from build123d import *

# Parameters (mm, degrees)
SKETCH1_W           = 30
SKETCH1_H           = 5
BOSS_EXTRUDE1_DEPTH = 15
SKETCH3_R           = 1
CUT_EXTRUDE2_DEPTH  = 5
SKETCH4_R           = 2
CUT_EXTRUDE3_DEPTH  = 1.5
SKETCH5_W           = 5
SKETCH5_H           = 10
BOSS_EXTRUDE2_DEPTH = 3


with BuildPart() as part:
    # Sketch1 → Boss-Extrude1 (new body)
    with BuildSketch(Plane(origin=(0, 0, 0), x_dir=(1, 0, 0), z_dir=(0, 1, 0))):
        with Locations((-41.880536913, 26.290268456)):
            Rectangle(SKETCH1_W, SKETCH1_H)
    extrude(amount=BOSS_EXTRUDE1_DEPTH)

    # Sketch3 → Cut-Extrude2 (cut)
    with BuildSketch(Plane(origin=(0, 0, -28.790268456), x_dir=(-1, 0, 0), z_dir=(0, 0, -1))):
        with Locations((35.880536913, 7.5)):
            Circle(SKETCH3_R)
        with Locations((32.880536913, 7.5)):
            Circle(SKETCH3_R)
        with Locations((29.880536913, 7.5)):
            Circle(SKETCH3_R)
        with Locations((53.880536913, 7.5)):
            Circle(SKETCH3_R)
        with Locations((50.880536913, 7.5)):
            Circle(SKETCH3_R)
        with Locations((47.880536913, 7.5)):
            Circle(SKETCH3_R)
    extrude(amount=-CUT_EXTRUDE2_DEPTH, mode=Mode.SUBTRACT)

    # Sketch4 → Cut-Extrude3 (cut)
    with BuildSketch(Plane(origin=(0, 0, -28.790268456), x_dir=(-1, 0, 0), z_dir=(0, 0, -1))):
        with Locations((41.880536913, 7.5)):
            Circle(SKETCH4_R)
    extrude(amount=-CUT_EXTRUDE3_DEPTH, mode=Mode.SUBTRACT)

    # Sketch5 → Boss-Extrude2 (add)
    with BuildSketch(Plane.XY.offset(-23.790268456)):
        with Locations((-59.380536913, 7.5)):
            Rectangle(SKETCH5_W, SKETCH5_H)
        with Locations((-24.380536913, 7.5)):
            Rectangle(SKETCH5_W, SKETCH5_H)
    extrude(amount=-BOSS_EXTRUDE2_DEPTH)


solid = part.part
Model file for the job. Use its own axes, mm. A direction names the side the tool comes from. Give positions to 0.01 mm unless a question says otherwise; leave off trailing zeros. Loops run counter-clockwise (first coordinate to the right, second up) from the corner with the lowest first, then second, coordinate; pieces in that order, holes last. Notation, with made-up numbers: (23.25, -26) - (28.25, -26) arc R20 ccw to (28.25, -2) - close; hole circle Ø11 at (-19, 58). An arc over 180 degrees is marked (long way). Use one line per item in the form item = value.
(1) Cut at C-C (y = 3.75). Give the cut face in (x, z), then the cut area to 3 significant figures.
Determined:
outline = (-61.88, -26.79) - (-56.88, -26.79) - (-56.88, -28.79) - (-26.88, -28.79) - (-26.88, -26.79) - (-21.88, -26.79) - (-21.88, -23.79) - (-61.88, -23.79) - close
area = 180 mm^2
(2) Drill centre lines: L1, parallel to X at y = 11.5, z = -27.2; L2, parallel to Y at x = -26, z = -25.1; L3, parallel to Z at x = -57.5, y = 6.5. Where is each one in solid material? Low to high.
Determined:
L1 = -56.88 to -26.88
L2 = 2.5 to 12.5
L3 = -26.79 to -23.79
(3) Pull direction Y, two halves, no side cores. Call faces 1 (the face through (-24, 2.5, -25)), 2 (the face through (-43.79, 8.1, -28.05)), 3 (the face through (-45, 7, -28.79)), 4 (the face through (-49.88, 7.54, -26.33)): pulls with the +Y half, pulls with the -Y half, needs draft (parallel to the pull), parting line crosses it, or undercut.
Determined:
face_1 = pulls with the -Y half
face_2 = undercut
face_3 = needs draft
face_4 = undercut
(4) Cut at D-D (y = 7.5). Count the separate pieces of the cut face and the enclosed holes in it, then the cut area to 3 significant figures.
Determined:
separate_pieces = 7
enclosed_holes = 0
area = 114 mm^2
(5) Cut at B-B (x = -53.5). Give the cut face in (y, z), then the cut area to 3 significant figures.
Determined:
outline = (0, -28.79) - (6.58, -28.79) - (6.58, -23.79) - (0, -23.79) - close; (8.42, -28.79) - (15, -28.79) - (15, -23.79) - (8.42, -23.79) - close
area = 65.8 mm^2
(6) Drop flat-ended pins along their axis: P1, Ø1.5, axis at x = -24.5, z = -25.5, coming from the -Y side; P2, Ø2.5, axis at x = -60, z = -25, coming from the +Y side; P3, Ø1.2, axis at x = -32.88, y = 7.5, coming from the -Z side; P4, Ø1.5, axis at x = -24.5, y = 9.5, coming from the -Z side. Give the stop position or say it passes through.
Determined:
P1 = 2.5
P2 = 12.5
P3 = through
P4 = -26.79
(7) 3-axis set-ups, long thin cutter, end or side, ignore diameter. For faces 5 (the face through (-59, 2.5, -25)), 6 (the face through (-24, 12.5, -25)), 7 (the face through (-59, 12.5, -25)), 8 (the face through (-24, 8, -26.79)), 9 (the face through (-59, 8, -26.79)): which of +Z, -Z, +X, -X, +Y, -Y reach the whole face in a straight line?
Determined:
face_5 = +Z, -Z, -X, -Y
face_6 = +Z, -Z, +X, +Y
face_7 = +Z, -Z, -X, +Y
face_8 = -Z, +X, +Y, -Y
face_9 = -Z, -X, +Y, -Y
(8) Cut at A-A (z = -25.8). Give the cut face in (x, y), then the cut area to 3 significant figures.
Determined:
outline = (-61.88, 2.5) - (-56.88, 2.5) - (-56.88, 0) - (-26.88, 0) - (-26.88, 2.5) - (-21.88, 2.5) - (-21.88, 12.5) - (-26.88, 12.5) - (-26.88, 15) - (-56.88, 15) - (-56.88, 12.5) - (-61.88, 12.5) - close; hole circle Ø2 at (-53.88, 7.5); hole circle Ø2 at (-50.88, 7.5); hole circle Ø2 at (-47.88, 7.5); hole circle Ø2 at (-35.88, 7.5); hole circle Ø2 at (-32.88, 7.5); hole circle Ø2 at (-29.88, 7.5)
area = 531 mm^2
